Build history of the part. All positions in model axes, mm. A direction names the side the tool comes from. Give positions to 0.01 mm unless a question says otherwise; leave off trailing zeros. Order: outer loops, then holes, each group sorted by start corner. A loop starts at its lowest first (then second) coordinate and runs counter-clockwise, first axis right, second up. Notation, with made-up numbers: (68.5, 68.25) -> (120.5, 68.25) arc R16 ccw to (120.5, 72.25) -> close; hole circle Ø8 at (-9, -24). An arc over 180 degrees is marked (long way). One line per item, written item: value. Start each with the question number.
(1) Saw through at B-B on x = 0. Give the cut face in (y, z), plus the area to 3 significant figures.
(2) Probe line 1 (X direction, y = 0, z = 0.5); line 2 (Y direction, x = 1.5, z = 1.05). List the from-to ranges inside material, lowest first.
(3) Pin check, flat tips, straight feed: pin 1 (1.6 mm diameter, centred on y = -22.5, z = 1.5, fed in from -X); pin 2 (1.6 mm diameter, centred on y = -21, z = 2.5, fed in from +X); pin 3 (0.8 mm diameter, centred on y = -21.5, z = -0.5, fed in from +X). Stop position of each tip, or through.
(4) Saw through at D-D on x = 21. Give the cut face in (y, z).
(5) Saw through at A-A on y = 0. Give the cut face in (x, z).
(6) Saw through at C-C on z = 1.85. Count the separate pieces of the cut face and the enclosed holes in it, plus the area to 3 significant figures.
(7) Two-plate mould, pull along Y, no slides. Class faces 5 (the flat face through (20.767, -12.03, 1.986)), 6 (the flat face through (21, -2.5, 2)), 7 (the flat face through (-2.5, 21, 2)): +Y half, -Y half, draft (parallel to the pull), parting line (faces both ways), or undercut.
(8) Which spindle directions (+Z, -Z, +X, -X, +Y, -Y) get a long thin tool onto all of the face, cutting with end or side? Do faces 1 (the flat face through (0, -19, 2)), 2 (the flat face through (-17.34, 12.9, 1.99)), 3 (the flat face through (21, 2.5, 2)), 4 (the flat face through (8.57, -19.84, 1.99)). Say none if no direction does.
```python
from build123d import *

# Parameters (mm, degrees)
SKIZZE1_R                       = 25.5
SKIZZE1_R_2                     = 17.5
AUFSATZ_LINEAR_AUSTRAGEN1_DEPTH = 1
AUFSATZ_LINEAR_AUSTRAGEN2_DEPTH = 1
SKIZZE3_W                       = 5
SKIZZE3_H                       = 5
AUFSATZ_LINEAR_AUSTRAGEN3_DEPTH = 2


with BuildPart() as part:
    # Skizze1 → Aufsatz-Linear austragen1 (new body)
    with BuildSketch(Plane.XY):
        Circle(SKIZZE1_R)
        Circle(SKIZZE1_R_2, mode=Mode.SUBTRACT)
    extrude(amount=AUFSATZ_LINEAR_AUSTRAGEN1_DEPTH)

    # Skizze2 → Aufsatz-Linear austragen2 (add)
    with BuildSketch(Plane(origin=(0, 0, 0), x_dir=(-1, 0, 0), z_dir=(0, 0, -1))):
        with BuildLine():
            Line((-6, -16.439282223), (-6, -24.784067463))
            ThreePointArc((-6, -24.784067463), (0, -25.5), (6, -24.784067463))
            Line((6, -24.784067463), (6, -16.439282223))
            ThreePointArc((6, -16.439282223), (0, -17.5), (-6, -16.439282223))
        make_face()
    extrude(amount=AUFSATZ_LINEAR_AUSTRAGEN2_DEPTH)

    # Skizze3 → Aufsatz-Linear austragen3 (add)
    with BuildSketch(Plane.XY.offset(1)):
        Polygon((-11.665063509, -15.204482672), (-14.165063509, -19.534609691), (-9.834936491, -22.034609691), (-7.334936491, -17.704482672), align=None)
        with Locations((0, -21.5)):
            Rectangle(SKIZZE3_W, SKIZZE3_H)
        Polygon((-17.704482672, -7.334936491), (-22.034609691, -9.834936491), (-19.534609691, -14.165063509), (-15.204482672, -11.665063509), align=None)
        with Locations((-21.5, 0)):
            Rectangle(SKIZZE3_W, SKIZZE3_H)
        Polygon((-15.204482672, 11.665063509), (-19.534609691, 14.165063509), (-22.034609691, 9.834936491), (-17.704482672, 7.334936491), align=None)
        Polygon((-7.334936491, 17.704482672), (-9.834936491, 22.034609691), (-14.165063509, 19.534609691), (-11.665063509, 15.204482672), align=None)
        with Locations((0, 21.5)):
            Rectangle(SKIZZE3_W, SKIZZE3_H)
        Polygon((11.665063509, 15.204482672), (14.165063509, 19.534609691), (9.834936491, 22.034609691), (7.334936491, 17.704482672), align=None)
        Polygon((17.704482672, 7.334936491), (22.034609691, 9.834936491), (19.534609691, 14.165063509), (15.204482672, 11.665063509), align=None)
        with Locations((21.5, 0)):
            Rectangle(SKIZZE3_W, SKIZZE3_H)
        Polygon((15.204482672, -11.665063509), (19.534609691, -14.165063509), (22.034609691, -9.834936491), (17.704482672, -7.334936491), align=None)
        Polygon((7.334936491, -17.704482672), (9.834936491, -22.034609691), (14.165063509, -19.534609691), (11.665063509, -15.204482672), align=None)
    extrude(amount=AUFSATZ_LINEAR_AUSTRAGEN3_DEPTH)


solid = part.part
```
Results below:
1. outline: (-25.5, -1) -> (-17.5, -1) -> (-17.5, 1) -> (-19, 1) -> (-19, 3) -> (-24, 3) -> (-24, 1) -> (-25.5, 1) -> close; (17.5, 0) -> (25.5, 0) -> (25.5, 1) -> (24, 1) -> (24, 3) -> (19, 3) -> (19, 1) -> (17.5, 1) -> close
1. area: 44.0 mm²
2. line 1: x = -25.5 to -17.5, 17.5 to 25.5
2. line 2: y = -24 to -19, 19 to 24
3. pin 1: stops at x = -13.1
3. pin 2: stops at x = 13.01
3. pin 3: stops at x = 6
4. outline: (-14.47, 0) -> (14.47, 0) -> (14.47, 1) -> (11.63, 1) -> (11.63, 3) -> (9.24, 3) -> (9.24, 1) -> (2.5, 1) -> (2.5, 3) -> (-2.5, 3) -> (-2.5, 1) -> (-9.24, 1) -> (-9.24, 3) -> (-11.63, 3) -> (-11.63, 1) -> (-14.47, 1) -> close
5. outline: (-25.5, 0) -> (-17.5, 0) -> (-17.5, 1) -> (-19, 1) -> (-19, 3) -> (-24, 3) -> (-24, 1) -> (-25.5, 1) -> close; (17.5, 0) -> (25.5, 0) -> (25.5, 1) -> (24, 1) -> (24, 3) -> (19, 3) -> (19, 1) -> (17.5, 1) -> close
6. separate pieces: 12
6. enclosed holes: 0
6. area: 300 mm²
7. face 5: -Y half
7. face 6: undercut
7. face 7: draft
8. face 1: +Z
8. face 2: +Z, +Y
8. face 3: +Z, +X, -X
8. face 4: +Z, -Y
